```python
from build123d import *

# Parameters (mm, degrees)
F0_R     = 7.9375
F0_R_2   = 11.43
F1_DEPTH = 4.7625


with BuildPart() as f1:
    # F0 (on Front) → F1 (new body)
    with BuildSketch(Plane.XZ):
        with BuildLine():
            Line((30.120686, 57.15), (19.00762, 57.15))
            Line((19.00762, 57.15), (19.00762, 33.02))
            ThreePointArc((19.00762, 33.02), (31.640757, -21.224337), (-23.341394, -30.112943))
            Line((-23.341394, -30.112943), (-82.945339, -133.350004))
            Line((-82.945339, -133.350004), (-36.502154, -133.350004))
            ThreePointArc((-36.502154, -133.350004), (-33.327154, -132.499265), (-31.002893, -130.175004))
            Line((-31.002893, -130.175004), (-9.005846, -92.075))
            ThreePointArc((-9.005846, -92.075), (-6.681584, -89.750739), (-3.506584, -88.9))
            Line((-3.506584, -88.9), (23.770686, -88.9))
            ThreePointArc((23.770686, -88.9), (28.260814, -90.759872), (30.120686, -95.25))
            ThreePointArc((30.120686, -95.25), (55.520686, -120.65), (80.920686, -95.25))
            Line((80.920686, -95.25), (80.920686, 57.15))
            ThreePointArc((80.920686, 57.15), (55.520686, 82.55), (30.120686, 57.15))
        make_face()
        with Locations((55.520686, -95.25)):
            Circle(F0_R, mode=Mode.SUBTRACT)
        with Locations((55.520686, -19.05)):
            Circle(F0_R_2, mode=Mode.SUBTRACT)
        with Locations((55.520686, 57.15)):
            Circle(F0_R, mode=Mode.SUBTRACT)
    extrude(amount=F1_DEPTH)


solid = f1.part
```
Geometry check sheet. Reference: the model listing, model coordinates, mm. A direction names the side the tool comes from. Coordinates: 2 decimals unless noted, no trailing zeros. Loops run counter-clockwise (first coordinate to the right, second up) from the corner with the lowest first, then second, coordinate; pieces in that order, holes last.
Item 1: Sectioned sample at A-A, the plane z = -35. Record the boundary of the cut face in (x, y).
Item 2: Release check for a two-part mould opening along Z. For faces 1 (the face through (32.12, -2.35, -20.49)), 2 (the face through (49.67, -2.348, 62.515)), 3 (the face through (16, -4.762, -48)), 4 (the face through (28.2, -2.3, -90.7)) record: released by +Z, released by -Z, zero draft, split by the parting line, or undercut.
Item 3: Sectioned sample at B-B, the plane x = 55. Record the boundary of the cut face in (y, z).
Item 4: Sectioned sample at C-C, the plane z = 0. Record the boundary of the cut face in (x, y).
Item 5: Thickness scan on line 1 (X direction, y = -4.35, z = -96); line 2 (X direction, y = -1.25, z = -81); line 3 (Z direction, x = -6, y = -3.9). Record the ranges inside material, lowest first.
Item 6: Go/stop test with flat-tipped pins: pin 1 Ø1.5 at (x, y) = (-19, -1) entering from +Z; pin 2 Ø20.5 at (x, z) = (55.52, -19.05) entering from -Y; pin 3 Ø2 at (x, y) = (-37, -3) entering from +Z; pin 4 Ø1.4 at (x, y) = (10, -2.5) entering from -Z. Record where each tip stops, or that it passes through.
Item 7: Sectioned sample at D-D, the plane x = 0. Record the boundary of the cut face in (y, z).
Item 8: Access from +Z, -Z, +X, -X, +Y, -Y to the whole of each face (thin tool, end or side, straight path). Record for faces 5 (the face through (10, -2, -88.9)), 6 (the face through (80.921, -2, -20)), 7 (the face through (25, -2, 57.15)).
Check result:
1. outline: (-26.16, -4.76) - (-15.05, -4.76) - (-15.05, 0) - (-26.16, 0) - close; (15.05, -4.76) - (80.92, -4.76) - (80.92, 0) - (15.05, 0) - close
2. face 1: undercut
2. face 2: undercut
2. face 3: zero draft
2. face 4: released by -Z
3. outline: (-4.76, -120.64) - (0, -120.64) - (0, -103.17) - (-4.76, -103.17) - close; (-4.76, -87.33) - (0, -87.33) - (0, -30.47) - (-4.76, -30.47) - close; (-4.76, -7.63) - (0, -7.63) - (0, 49.23) - (-4.76, 49.23) - close; (-4.76, 65.07) - (0, 65.07) - (0, 82.54) - (-4.76, 82.54) - close
4. outline: (38.1, -4.76) - (80.92, -4.76) - (80.92, 0) - (38.1, 0) - close
5. line 1: x = -61.38 to -11.27, 30.13 to 47.62, 63.42 to 80.91
5. line 2: x = -52.72 to 80.92
5. line 3: z = -89.41 to -37.62
6. pin 1: stops at z = -32.58
6. pin 2: passes through
6. pin 3: stops at z = -52.04
6. pin 4: stops at z = -88.9
7. outline: (-4.76, -88.9) - (0, -88.9) - (0, -38.1) - (-4.76, -38.1) - close
8. face 5: -Z, +Y, -Y
8. face 6: +Z, -Z, +X, +Y, -Y
8. face 7: +Z, -X, +Y, -Y
